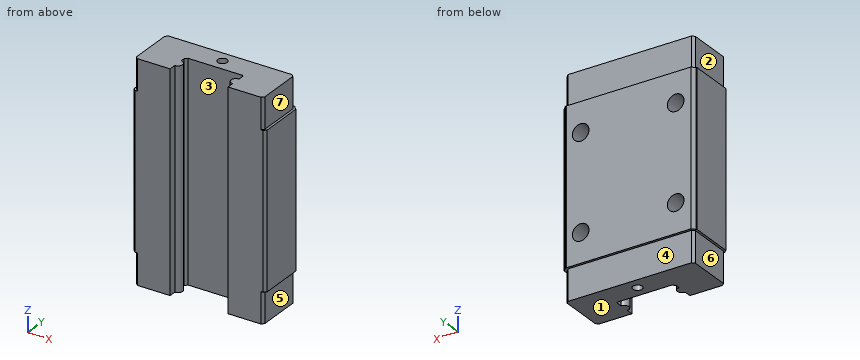
```python
from build123d import *
from build123d.topology import SkipClean

# Parameters (mm, degrees)
SKETCH1_R                 = 1
BOSS_EXTRUDE1_DEPTH       = 45.4
BOSS_EXTRUDE2_START       = -38.9
SKETCH5_R                 = 1
BOSS_EXTRUDE2_DEPTH       = 32.4
M5X0_8_TAPPED_HOLE1_D     = 3.5
M5X0_8_TAPPED_HOLE1_DEPTH = 4
M5X0_8_TAPPED_HOLE1_TIP   = 1.051506083


with BuildPart() as part:
    # Sketch1 → Boss-Extrude1 (new body)
    with BuildSketch(Plane.XY):
        with BuildLine():
            Line((-13.5, -4.5), (-13, -5))
            Line((-13, -5), (-6.1, -5))
            Line((-6.1, -5), (-6.1, -3.5))
            ThreePointArc((-6.1, -3.5), (-5.1, -2.5), (-6.1, -1.5))
            Line((-6.1, -1.5), (-6.1, -0.5))
            Line((-6.1, -0.5), (-5.6, 0))
            Line((-5.6, 0), (5.85, 0))
            Line((5.85, 0), (6.1, -0.25))
            Line((6.1, -0.25), (6.1, -1.5))
            ThreePointArc((6.1, -1.5), (5.1, -2.5), (6.1, -3.5))
            Line((6.1, -3.5), (6.1, -5))
            Line((6.1, -5), (13, -5))
            Line((13, -5), (13.5, -4.5))
            Line((13.5, -4.5), (13.5, 4.5))
            Line((13.5, 4.5), (13, 5))
            Line((13, 5), (-13, 5))
            Line((-13, 5), (-13.5, 4.5))
            Line((-13.5, 4.5), (-13.5, -4.5))
        make_face()
        with Locations((0, 2.5)):
            Circle(SKETCH1_R, mode=Mode.SUBTRACT)
    extrude(amount=BOSS_EXTRUDE1_DEPTH)

    # Sketch5 → Boss-Extrude2 (add)
    with SkipClean():  # the faces are left unmerged after this step: merging them gives an invalid solid
        with BuildSketch(Plane.XY.offset(45.4).offset(BOSS_EXTRUDE2_START)):
            with BuildLine():
                Line((13, 5.5), (13.210808273, 5.496298508))
                Line((13.210808273, 5.496298508), (13.353553391, 5.353553391))
                Line((13.353553391, 5.353553391), (14, 4.707106781))
                Line((14, 4.707106781), (14, -4.5))
                Line((14, -4.5), (13.5, -5))
                Line((13.5, -5), (6.1, -5))
                Line((6.1, -5), (6.1, -3.5))
                ThreePointArc((6.1, -3.5), (5.1, -2.5), (6.1, -1.5))
                Line((6.1, -1.5), (6.1, -0.25))
                Line((6.1, -0.25), (5.85, 0))
                Line((5.85, 0), (-5.6, 0))
                Line((-5.6, 0), (-6.1, -0.5))
                Line((-6.1, -0.5), (-6.1, -1.5))
                ThreePointArc((-6.1, -1.5), (-5.1, -2.5), (-6.1, -3.5))
                Line((-6.1, -3.5), (-6.1, -5))
                Line((-6.1, -5), (-13.5, -5))
                Line((-13.5, -5), (-14, -4.5))
                Line((-14, -4.5), (-14, 4.5))
                Line((-14, 4.5), (-14, 4.707106781))
                Line((-14, 4.707106781), (-13.853553391, 4.853553391))
                Line((-13.853553391, 4.853553391), (-13.207106781, 5.5))
                Line((-13.207106781, 5.5), (13, 5.5))
            make_face()
            with Locations((0, 2.5)):
                Circle(SKETCH5_R, mode=Mode.SUBTRACT)
        extrude(amount=BOSS_EXTRUDE2_DEPTH)
    add(part.part.scale(1), mode=Mode.REPLACE)  # the faces are merged on a copy

    # M5x0.8 Tapped Hole1
    with Locations(Plane(origin=(0, 5.5, 0), x_dir=(1, 0, 0), z_dir=(0, 1, 0))):
        with Locations((-10, -12.7), (-10, -32.7), (10, -32.7), (10, -12.7)):
            Hole(M5X0_8_TAPPED_HOLE1_D / 2, depth=M5X0_8_TAPPED_HOLE1_DEPTH)
            with Locations((0, 0, -(M5X0_8_TAPPED_HOLE1_DEPTH + M5X0_8_TAPPED_HOLE1_TIP / 2))):  # 118° drill point
                Cone(0, M5X0_8_TAPPED_HOLE1_D / 2, M5X0_8_TAPPED_HOLE1_TIP, mode=Mode.SUBTRACT)


solid = part.part
```
Could you check a few things on this model? Use its own coordinates, in mm. Face numbers are marked on the shaded views. A direction names the side the tool comes from. Give positions to 0.01 mm unless a question says otherwise; leave off trailing zeros. Loops run counter-clockwise (first coordinate to the right, second up) from the corner with the lowest first, then second, coordinate; pieces in that order, holes last. Notation, with made-up numbers: (56.5, 70.5) - (112.5, 70.5) arc R23 ccw to (112.5, 101.5) - close; hole circle Ø5 at (74.25, 11). An arc over 180 degrees is marked (long way). Use one line per item in the form item = value.
1. On a 3-axis mill with a long thin cutter (end or side, diameter ignored), from which of +Z, -Z, +X, -X, +Y, -Y can I reach the whole of each face in a straight line? I mean the marked faces 4, 5, 6 and 7. Say none if no direction works.
Response values:
face_4 = -Z, +X, -X, +Y
face_5 = -Z, +X, +Y, -Y
face_6 = -Z, -X, +Y, -Y
face_7 = +Z, +X, +Y, -Y
2. I want a section at C-C (x = 0). Please give me the cut outline in (y, z).
Response values:
outline = (0, 0) - (1.5, 0) - (1.5, 45.4) - (0, 45.4) - close; (3.5, 0) - (5, 0) - (5, 6.5) - (5.5, 6.5) - (5.5, 38.9) - (5, 38.9) - (5, 45.4) - (3.5, 45.4) - close
3. I want a section at A-A (y = 2.5). Please give me the cut outline in (x, z), and give its area (3 significant figures).
Response values:
outline = (-14, 6.5) - (-13.5, 6.5) - (-13.5, 0) - (-1, 0) - (-1, 45.4) - (-13.5, 45.4) - (-13.5, 38.9) - (-14, 38.9) - close; (1, 0) - (13.5, 0) - (13.5, 6.5) - (14, 6.5) - (14, 38.9) - (13.5, 38.9) - (13.5, 45.4) - (1, 45.4) - close; hole circle Ø3.5 at (-10, 12.7); hole circle Ø3.5 at (-10, 32.7); hole circle Ø3.5 at (10, 12.7); hole circle Ø3.5 at (10, 32.7)
area = 1,130 mm²
4. I'm going to push flat-ended pins straight in: pin 1 Ø3 at (x, y) = (3, -0.5) entering from +Z; pin 2 Ø3 at (x, z) = (0, 2.5) entering from +Y; pin 3 Ø2 at (x, z) = (10, 32.7) entering from +Y; pin 4 Ø2 at (y, z) = (-1.5, 4) entering from +X. Where does each tip first touch, or does it pass through?
Response values:
pin_1 = 45.4
pin_2 = 5
pin_3 = 1.05
pin_4 = 13.5
5. I need wall thicknesses on probe 1 along X at (y, z) = (3.6, 12.7); probe 2 along Z at (x, y) = (10, 2.4); probe 3 along X at (y, z) = (-1, 16). Which ranges of each line are inside material? Lowest first, please.
Response values:
probe_1 = -14 to -11.75, -8.25 to 8.25, 11.75 to 14
probe_2 = 0 to 10.95, 14.45 to 30.95, 34.45 to 45.4
probe_3 = -14 to -6.1, 6.1 to 14
6. I want a section at B-B (z = 5). Please give me the cut outline in (x, y).
Response values:
outline = (-13.5, -4.5) - (-13, -5) - (-6.1, -5) - (-6.1, -3.5) arc R1 ccw to (-6.1, -1.5) - (-6.1, -0.5) - (-5.6, 0) - (5.85, 0) - (6.1, -0.25) - (6.1, -1.5) arc R1 ccw to (6.1, -3.5) - (6.1, -5) - (13, -5) - (13.5, -4.5) - (13.5, 4.5) - (13, 5) - (-13, 5) - (-13.5, 4.5) - close; hole circle Ø2 at (0, 2.5)
7. Thinking about a two-plate mould opening in X: for the marked faces 1, 2 and 3, which applies, released by +X, released by -X, zero draft, split by the parting line, or undercut?
Response values:
face_1 = zero draft
face_2 = released by -X
face_3 = undercut
8. I want a section at D-D (y = -2.5). Please give me the cut outline in (x, z), and give its area (3 significant figures).
Response values:
outline = (-14, 6.5) - (-13.5, 6.5) - (-13.5, 0) - (-5.1, 0) - (-5.1, 45.4) - (-13.5, 45.4) - (-13.5, 38.9) - (-14, 38.9) - close; (5.1, 0) - (13.5, 0) - (13.5, 6.5) - (14, 6.5) - (14, 38.9) - (13.5, 38.9) - (13.5, 45.4) - (5.1, 45.4) - close
area = 795 mm²
